```python
from build123d import *

# Parameters (mm, degrees)
F0_W          = 20
F0_H          = 25
F0_R          = 4.025
F1_DEPTH      = 12
F1_DEPTH_BACK = 12
F2_DEPTH      = 8.1
F2_DEPTH_BACK = 8.1
F3_R          = 3
F4_R          = 5
F6_D          = 8.4328
F6_DEPTH      = 30.794
F6_TIP        = 2.5334687141
F7_SIZE       = 2


with BuildPart() as f1:
    # F0 (on Front) → F1 (new body, two sides)
    with BuildSketch(Plane.XZ) as f1_sk:
        with Locations((10, 12.5)):
            Rectangle(F0_W, F0_H)
        with BuildLine():
            Line((20, 25), (20, 0))
            Line((20, 0), (50, 0))
            Line((50, 0), (50, 13))
            ThreePointArc((50, 13), (46.4852813742, 21.4852813742), (38, 25))
            Line((38, 25), (20, 25))
        make_face()
        with Locations((38, 13)):
            Circle(F0_R, mode=Mode.SUBTRACT)
    extrude(amount=F1_DEPTH)
    extrude(f1_sk.sketch, amount=-F1_DEPTH_BACK)

    # F0 (on Front) → F2 (cut, two sides)
    with BuildSketch(Plane.XZ) as f2_sk:
        with BuildLine():
            Line((20, 25), (20, 0))
            Line((20, 0), (50, 0))
            Line((50, 0), (50, 13))
            ThreePointArc((50, 13), (46.4852813742, 21.4852813742), (38, 25))
            Line((38, 25), (20, 25))
        make_face()
        with Locations((38, 13)):
            Circle(F0_R, mode=Mode.SUBTRACT)
    extrude(amount=-F2_DEPTH, mode=Mode.SUBTRACT)
    extrude(f2_sk.sketch, amount=F2_DEPTH_BACK, mode=Mode.SUBTRACT)

    # F3
    f3_edges = [f1.edges().sort_by_distance(p)[0] for p in [
        (20, -8.1, 12.5),
        (20, 8.1, 12.5),
    ]]
    fillet(f3_edges, radius=F3_R)

    # F4
    f4_edges = [f1.edges().sort_by_distance(p)[0] for p in [
        (50, -10.05, 0),
        (50, 10.05, 0),
    ]]
    fillet(f4_edges, radius=F4_R)

    # F6
    with Locations(Plane(origin=(0, 0, 0), x_dir=(0, -1, 0), z_dir=(-1, 0, 0))):
        with Locations((0, 13.2)):
            Hole(F6_D / 2, depth=F6_DEPTH)
            with Locations((0, 0, -(F6_DEPTH + F6_TIP / 2))):  # 118° drill point
                Cone(0, F6_D / 2, F6_TIP, mode=Mode.SUBTRACT)

    # F7
    f7_edges = [f1.edges().sort_by_distance(p)[0] for p in [
        (0, 0, 0),
    ]]
    chamfer(f7_edges, length=F7_SIZE)


solid = f1.part
```
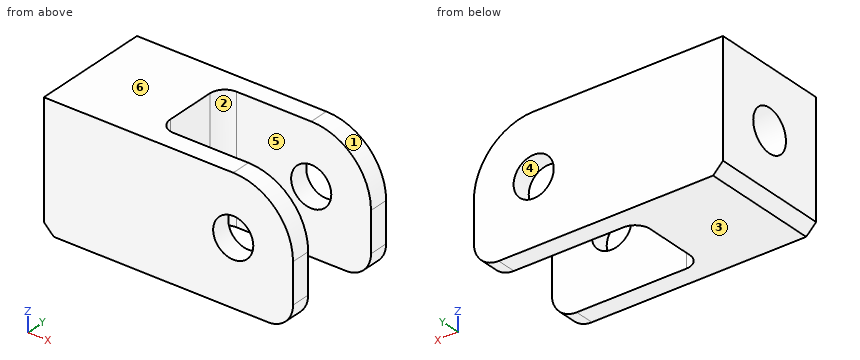
Here's how the part is built. I have some questions about the finished solid (model axes, mm). Face numbers are marked on the shaded views. A direction names the side the tool comes from. Give positions to 0.01 mm unless a question says otherwise; leave off trailing zeros. Write each loop counter-clockwise with the first axis right and the second up, starting at its lowest first coordinate (ties: lowest second). Pieces come first, ordered by that corner, then holes. Notation, with made-up numbers: M 17,-10.5 L 71,-10.5 A35 ccw 71,21.5 Z; hole C 16.5,-21 d2. An arc over 180 degrees is marked long. Put each result on its own line as item: value. Start each with the question number.
Item 1: Thinking about a two-plate mould opening in Z: for the marked faces 3, 4, 5 and 6, which applies, +Z half, -Z half, draft (parallel to the pull), parting line (faces both ways), or undercut?
Item 2: I need wall thicknesses on L1, parallel to Z at x = 12.75, y = 0; L2, parallel to Z at x = 38, y = -10.3 (3 decimals); L3, parallel to Y at x = 24, z = 4.5. Which ranges of each line are inside material? Lowest first, please. Write a range as from..to.
Item 3: If we section it at B-B, the plane x = 18.5: Write out the boundary of the cut face in (y, z), then the cut area to 3 significant figures.
Item 4: Will these pins go through, and if not, where does the flat tip stop? pin 1 (11 mm diameter, centred on y = -2, z = 13, fed in from +X); pin 2 (8 mm diameter, centred on y = 3, z = 22.5, fed in from +X); pin 3 (8 mm diameter, centred on x = 40.5, y = 1, fed in from +Z).
Item 5: If we section it at A-A, the plane y = 0: Write out the boundary of the cut face in (x, z).
Item 6: If we section it at D-D, the plane y = 7.5: Write out the boundary of the cut face in (x, z).
Item 7: On a 3-axis mill with a long thin cutter (end or side, diameter ignored), from which of +Z, -Z, +X, -X, +Y, -Y can I reach the whole of each face in a straight line? I mean the marked faces 1 and 2. Say none if no direction works.
Item 8: If we section it at C-C, the plane z = 10.5: Write out the boundary of the cut face in (x, y).
Values:
1. face 3: -Z half
1. face 4: undercut
1. face 5: draft
1. face 6: +Z half
2. L1: 0..8.98, 17.42..25
2. L2: 0..8.975, 17.025..25
2. L3: -12..-8.1, 8.1..12
3. outline: M -12,0 L 12,0 L 12,25 L -12,25 Z; hole C 0,13.2 d8.43
3. area: 544 mm²
4. pin 1: x = 21.2
4. pin 2: x = 20.68
4. pin 3: through
5. outline: M 0,2 L 2,0 L 20,0 L 20,8.98 L 0,8.98 Z; M 0,17.42 L 20,17.42 L 20,25 L 0,25 Z
6. outline: M 0,2 L 2,0 L 21.2,0 L 21.2,25 L 0,25 Z
7. face 1: +Z, +X, +Y, -Y
7. face 2: +Z, -Z, +X
8. outline: M 0,-12 L 34.85,-12 L 34.85,-8.1 L 23,-8.1 A3 cw 20,-5.1 L 20,-3.24 L 0,-3.24 Z; M 0,3.24 L 20,3.24 L 20,5.1 A3 cw 23,8.1 L 34.85,8.1 L 34.85,12 L 0,12 Z; M 41.15,-12 L 50,-12 L 50,-8.1 L 41.15,-8.1 Z; M 41.15,8.1 L 50,8.1 L 50,12 L 41.15,12 Z
